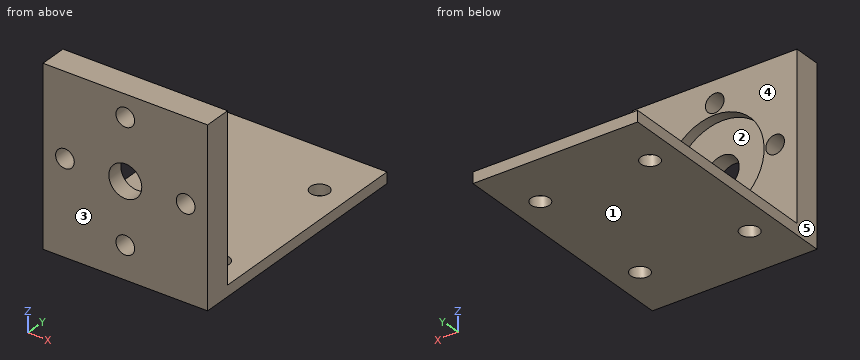
```python
from build123d import *

# Parameters (mm, degrees)
BOSS_EXTRUDE1_DEPTH     = 30
SKETCH3_R               = 9
SKETCH3_R_2             = 3
CUT_EXTRUDE1_DEPTH      = 2
SKETCH7_R               = 3
CUT_EXTRUDE2_DEPTH      = 60.363288319
CUT_EXTRUDE3_DEPTH      = 2
CUT_EXTRUDE3_DEPTH_BACK = 61.728905803
SKETCH8_R               = 1.7
SKETCH9_R               = 1.7
CUT_EXTRUDE4_DEPTH      = 62.846584384


with BuildPart() as part:
    # Sketch2 → Boss-Extrude1 (new body)
    with BuildSketch(Plane(origin=(0, 0, 0), x_dir=(0, 0, -1), z_dir=(1, 0, 0))):
        Polygon((0, 0), (32, 0), (32, 45), (30, 45), (30, 5), (0, 5), align=None)
    extrude(amount=BOSS_EXTRUDE1_DEPTH)

    # Sketch3 → Cut-Extrude1 (cut)
    with BuildSketch(Plane(origin=(0, 5, 0), x_dir=(1, 0, 0), z_dir=(0, 1, 0))):
        with Locations(Location((15, 15, 0), (0, 0, 270))):
            Circle(SKETCH3_R)
        with Locations(Location((15, 15, 0), (0, 0, 270))):
            Circle(SKETCH3_R_2, mode=Mode.SUBTRACT)
    extrude(amount=-CUT_EXTRUDE1_DEPTH, mode=Mode.SUBTRACT)

    # Sketch7 → Cut-Extrude2 (cut, through all)
    with BuildSketch(Plane(origin=(0, 5, 0), x_dir=(1, 0, 0), z_dir=(0, 1, 0))):
        with Locations(Location((15, 15, 0), (0, 0, 270))):
            Circle(SKETCH7_R)
    extrude(amount=-CUT_EXTRUDE2_DEPTH, mode=Mode.SUBTRACT)

    # Sketch8 → Cut-Extrude3 (cut, two sides: drawn at the far end of the back side and taken through both)
    with BuildSketch(Plane(origin=(0, 3, 0), x_dir=(1, 0, 0), z_dir=(0, 1, 0)).offset(-CUT_EXTRUDE3_DEPTH_BACK)):
        with Locations(Location((4, 15, 0), (0, 0, 270))):
            Circle(SKETCH8_R)
        with Locations(Location((26, 15, 0), (0, 0, 270))):
            Circle(SKETCH8_R)
        with Locations(Location((15, 4, 0), (0, 0, 270))):
            Circle(SKETCH8_R)
        with Locations(Location((15, 26, 0), (0, 0, 270))):
            Circle(SKETCH8_R)
    extrude(amount=CUT_EXTRUDE3_DEPTH + CUT_EXTRUDE3_DEPTH_BACK, mode=Mode.SUBTRACT)

    # Sketch9 → Cut-Extrude4 (cut, through all)
    with BuildSketch(Plane.XY.offset(-30)):
        with Locations((5, 35)):
            Circle(SKETCH9_R)
        with Locations((25, 35)):
            Circle(SKETCH9_R)
        with Locations((25, 10)):
            Circle(SKETCH9_R)
        with Locations((5, 10)):
            Circle(SKETCH9_R)
    extrude(amount=-CUT_EXTRUDE4_DEPTH, mode=Mode.SUBTRACT)


solid = part.part
```
Geometry check sheet. Reference: the model listing, model coordinates, mm. Face numbers are marked on the shaded views. A direction names the side the tool comes from. Give positions to 0.01 mm unless a question says otherwise; leave off trailing zeros. Order: outer loops, then holes, each group sorted by start corner. A loop starts at its lowest first (then second) coordinate and runs counter-clockwise, first axis right, second up. Notation, with made-up numbers: (35, 40.25) - (69, 40.25) arc R24 cw to (69, 52.25) - close; hole circle Ø8 at (-17.75, 2.5). An arc over 180 degrees is marked (long way). Write item = value, one per line. Start each with the question number.
1) Section check A-A (x = 25). Enter the section's corners in (y, z).
2) Section check B-B (z = -27). Enter the section's corners in (x, y), then the cut area to 3 significant figures.
3) Draft check along Z on the marked faces 1, 2 and 3. Enter one of: released by +Z, released by -Z, zero draft, split by the parting line, or undercut.
4) Access from +Z, -Z, +X, -X, +Y, -Y to the whole of each face (thin tool, end or side, straight path). Record for the marked faces 4 and 5.
5) Section check D-D (x = 19.75). Enter the section's corners in (y, z), then the cut area to 3 significant figures.
6) Gauge pin test, flat ends, axial feed: pin 1 Ø15 at (x, z) = (21, -11) entering from +Y; pin 2 Ø4.5 at (x, y) = (25, 10) entering from +Z. Record the tip position at first contact, or that the pin passes through.
7) Scan lines: L1, parallel to X at y = 1.6, z = -4; L2, parallel to Y at x = 5, z = -30.55; L3, parallel to Y at x = 20, z = -18.5. Record each from-to range of solid material in increasing order.
8) Section check C-C (x = 12.75). Enter the section's corners in (y, z), then the cut area to 3 significant figures.
Geometry check:
q1.outline = (0, -32) - (8.3, -32) - (8.3, -30) - (5, -30) - (5, -16.37) - (0, -16.37) - close; (0, -13.63) - (5, -13.63) - (5, 0) - (0, 0) - close; (11.7, -32) - (33.3, -32) - (33.3, -30) - (11.7, -30) - close; (36.7, -32) - (45, -32) - (45, -30) - (36.7, -30) - close
q2.outline = (0, 0) - (13.63, 0) - (13.63, 5) - (0, 5) - close; (16.37, 0) - (30, 0) - (30, 5) - (16.37, 5) - close
q2.area = 136 mm2
q3.face_1 = released by -Z
q3.face_2 = undercut
q3.face_3 = zero draft
q4.face_4 = +Z, +X, -X, +Y
q4.face_5 = +Z, -Z, -X, +Y, -Y
q5.outline = (0, -32) - (45, -32) - (45, -30) - (5, -30) - (5, -22.64) - (3, -22.64) - (3, -7.36) - (5, -7.36) - (5, 0) - (0, 0) - close
q5.area = 209 mm2
q6.pin_1 = 5
q6.pin_2 = -30
q7.L1 = 0 to 13.3, 16.7 to 30
q7.L2 = 0 to 8.3, 11.7 to 33.3, 36.7 to 45
q7.L3 = 0 to 3
q8.outline = (0, -32) - (45, -32) - (45, -30) - (5, -30) - (5, -23.71) - (3, -23.71) - (3, -16.98) - (0, -16.98) - close; (0, -13.02) - (3, -13.02) - (3, -6.29) - (5, -6.29) - (5, 0) - (0, 0) - close
q8.area = 193 mm2
